Verification items for the finished model (mm, model axes). Give positions to 0.01 mm unless a question says otherwise; leave off trailing zeros. Write each loop counter-clockwise with the first axis right and the second up, starting at its lowest first coordinate (ties: lowest second). Pieces come first, ordered by that corner, then holes. Notation, with made-up numbers: (10, 24) -> (57, 24) arc R25 ccw to (57, 52) -> close; hole circle Ø7 at (8.25, 58). An arc over 180 degrees is marked (long way). Answer as CSV lines item,"result".
```python
from build123d import *

# Parameters (mm, degrees)
BOSS_EXTRUDE1_DEPTH = 6
CUT_EXTRUDE2_DEPTH  = 6
SKETCH4_R           = 1.6
SKETCH4_W           = 18
SKETCH4_H           = 12
CUT_EXTRUDE3_DEPTH  = 10
FILLET1_R           = 2
FILLET2_R           = 2
SKETCH5_R           = 1.1
CUT_EXTRUDE4_DEPTH  = 10
SKETCH6_R           = 22.5
CUT_EXTRUDE5_DEPTH  = 10
FILLET4_R           = 10
FILLET5_R           = 10
FILLET6_R           = 10
FILLET7_R           = 10
FILLET8_R           = 3
SKETCH8_W           = 40
SKETCH8_H           = 10
CUT_EXTRUDE11_DEPTH = 10
FILLET9_R           = 5
CUT_EXTRUDE13_DEPTH = 10
FILLET10_R          = 2


with BuildPart() as part:
    # Sketch1 → Boss-Extrude1 (new body)
    with BuildSketch(Plane.XY):
        Polygon((0, -126.72), (0, 0), (-109.742739168, 63.36), (-137.242739168, 15.728602792), (-55, -126.72), align=None)
        Polygon((-109.742739168, 63.36), (0, 0), (100, 57.735026919), (109.742739168, 63.36), (82.242739168, 110.991397208), (-82.242739168, 110.991397208), align=None)
        Polygon((100, 57.735026919), (0, 0), (0, -126.72), (55, -126.72), (137.242739168, 15.728602792), (109.742739168, 63.36), align=None)
    extrude(amount=BOSS_EXTRUDE1_DEPTH)

    # Sketch3 → Cut-Extrude2 (cut)
    with BuildSketch(Plane.XY.offset(6)):
        Polygon((-109.742739168, 63.36), (-114.742739168, 54.699745962), (-62.78121494, 24.699745962), (-57.78121494, 33.36), align=None)
        Polygon((-104.742739168, 72.020254038), (-109.742739168, 63.36), (-57.78121494, 33.36), (-52.78121494, 42.020254038), align=None)
        Polygon((104.742739168, 72.020254038), (52.78121494, 42.020254038), (57.78121494, 33.36), (62.78121494, 24.699745962), (114.742739168, 54.699745962), align=None)
        Polygon((10, -126.72), (10, -66.72), (0, -66.72), (-10, -66.72), (-10, -126.72), align=None)
    extrude(amount=-CUT_EXTRUDE2_DEPTH, mode=Mode.SUBTRACT)

    # Sketch4 → Cut-Extrude3 (cut)
    with BuildSketch(Plane.XY.offset(6)):
        with Locations((21, -87.47)):
            Circle(SKETCH4_R)
        with Locations((33, -87.47)):
            Circle(SKETCH4_R)
        with Locations((21, -111.47)):
            Circle(SKETCH4_R)
        with Locations((33, -111.47)):
            Circle(SKETCH4_R)
        with Locations((-86.251242069, 25.548466521)):
            Circle(SKETCH4_R)
        with Locations((-92.251242069, 15.156161675)):
            Circle(SKETCH4_R)
        with Locations((-113.03585176, 27.156161675)):
            Circle(SKETCH4_R)
        with Locations((-107.03585176, 37.548466521)):
            Circle(SKETCH4_R)
        with Locations((65.251242069, 61.921533479)):
            Circle(SKETCH4_R)
        with Locations((59.251242069, 72.313838325)):
            Circle(SKETCH4_R)
        with Locations((80.03585176, 84.313838325)):
            Circle(SKETCH4_R)
        with Locations((86.03585176, 73.921533479)):
            Circle(SKETCH4_R)
        Polygon((-111.856909844, 25.898148973), (-101.464604998, 19.898148973), (-110.464604998, 4.309691705), (-120.856909844, 10.309691705), align=None)
        Polygon((69.356909844, 99.510308295), (58.964604998, 93.510308295), (67.964604998, 77.921851027), (78.356909844, 83.921851027), align=None)
        with Locations((42.5, -103.82)):
            Rectangle(SKETCH4_W, SKETCH4_H)
    extrude(amount=-CUT_EXTRUDE3_DEPTH, mode=Mode.SUBTRACT)

    # Fillet1
    fillet1_edges = [part.edges().sort_by_distance(p)[0] for p in [
        (33.5, -109.82, 3),
        (33.5, -97.82, 3),
        (51.5, -97.82, 3),
        (51.5, -109.82, 3),
    ]]
    fillet(fillet1_edges, radius=FILLET1_R)

    # Fillet2
    fillet2_edges = [part.edges().sort_by_distance(p)[0] for p in [
        (-120.856909844, 10.309691705, 3),
        (-111.856909844, 25.898148973, 3),
        (-101.464604998, 19.898148973, 3),
        (-110.464604998, 4.309691705, 3),
    ]]
    fillet(fillet2_edges, radius=FILLET2_R)

    # Sketch5 → Cut-Extrude4 (cut)
    with BuildSketch(Plane.XY.offset(6)):
        with Locations((115.495143903, 45.896542732)):
            Circle(SKETCH5_R)
        with Locations((108.999953375, 42.146542732)):
            Circle(SKETCH5_R)
        with Locations((102.504762847, 38.396542732)):
            Circle(SKETCH5_R)
        with Locations((-18, -122.97)):
            Circle(SKETCH5_R)
        with Locations((-18, -115.47)):
            Circle(SKETCH5_R)
        with Locations((-18, -107.97)):
            Circle(SKETCH5_R)
        with Locations((-97.495143903, 77.073457268)):
            Circle(SKETCH5_R)
        with Locations((-90.999953375, 73.323457268)):
            Circle(SKETCH5_R)
        with Locations((-84.504762847, 69.573457268)):
            Circle(SKETCH5_R)
    extrude(amount=-CUT_EXTRUDE4_DEPTH, mode=Mode.SUBTRACT)

    # Sketch6 → Cut-Extrude5 (cut)
    with BuildSketch(Plane.XY.offset(6)):
        Circle(SKETCH6_R)
    extrude(amount=-CUT_EXTRUDE5_DEPTH, mode=Mode.SUBTRACT)

    # Fillet4
    fillet4_edges = [part.edges().sort_by_distance(p)[0] for p in [
        (-10, -66.72, 3),
        (10, -66.72, 3),
    ]]
    fillet(fillet4_edges, radius=FILLET4_R - 0.0001)  # a hair under: the kernel refuses the full size

    # Fillet5
    fillet5_edges = [part.edges().sort_by_distance(p)[0] for p in [
        (62.78121494, 24.699745962, 3),
        (52.78121494, 42.020254038, 3),
    ]]
    fillet(fillet5_edges, radius=FILLET5_R - 0.0001)  # a hair under: the kernel refuses the full size

    # Fillet6
    fillet6_edges = [part.edges().sort_by_distance(p)[0] for p in [
        (-52.78121494, 42.020254038, 3),
        (-62.78121494, 24.699745962, 3),
    ]]
    fillet(fillet6_edges, radius=FILLET6_R - 0.0001)  # a hair under: the kernel refuses the full size

    # Fillet7
    fillet7_edges = [part.edges().sort_by_distance(p)[0] for p in [
        (55, -126.72, 3),
        (-55, -126.72, 3),
        (-137.242739168, 15.728602792, 3),
        (-82.242739168, 110.991397208, 3),
        (82.242739168, 110.991397208, 3),
        (137.242739168, 15.728602792, 3),
    ]]
    fillet(fillet7_edges, radius=FILLET7_R)

    # Fillet8
    fillet8_edges = [part.edges().sort_by_distance(p)[0] for p in [
        (-114.742739168, 54.699745962, 3),
        (-104.742739168, 72.020254038, 3),
        (104.742739168, 72.020254038, 3),
        (114.742739168, 54.699745962, 3),
        (10, -126.72, 3),
        (-10, -126.72, 3),
    ]]
    fillet(fillet8_edges, radius=FILLET8_R)

    # Sketch8 → Cut-Extrude11 (cut)
    with BuildSketch(Plane.XY.offset(6)):
        with Locations((0, 35)):
            Rectangle(SKETCH8_W, SKETCH8_H)
        with Locations((0, -35)):
            Rectangle(SKETCH8_W, SKETCH8_H)
    extrude(amount=-CUT_EXTRUDE11_DEPTH, mode=Mode.SUBTRACT)

    # Fillet9
    fillet9_edges = [part.edges().sort_by_distance(p)[0] for p in [
        (20, -40, 3),
        (20, -30, 3),
        (-20, -40, 3),
        (-20, -30, 3),
        (20, 30, 3),
        (20, 40, 3),
        (-20, 30, 3),
        (-20, 40, 3),
    ]]
    fillet(fillet9_edges, radius=FILLET9_R - 0.0001)  # a hair under: the kernel refuses the full size

    # Sketch7 → Cut-Extrude13 (cut)
    with BuildSketch(Plane.XY.offset(6)):
        with BuildLine():
            Line((-47.1, 80), (-47.1, -80))
            ThreePointArc((-47.1, -80), (-45, -82.1), (-42.9, -80))
            Line((-42.9, -80), (-42.9, 80))
            ThreePointArc((-42.9, 80), (-45, 82.1), (-47.1, 80))
        make_face()
        with BuildLine():
            Line((42.9, 80), (42.9, -80))
            ThreePointArc((42.9, -80), (45, -82.1), (47.1, -80))
            Line((47.1, -80), (47.1, 80))
            ThreePointArc((47.1, 80), (45, 82.1), (42.9, 80))
        make_face()
        with BuildLine():
            Line((-105, 2.1), (-65, 2.1))
            ThreePointArc((-65, 2.1), (-62.9, 0), (-65, -2.1))
            Line((-65, -2.1), (-105, -2.1))
            ThreePointArc((-105, -2.1), (-107.1, 0), (-105, 2.1))
        make_face()
        with BuildLine():
            Line((65, 2.1), (105, 2.1))
            ThreePointArc((105, 2.1), (107.1, 0), (105, -2.1))
            Line((105, -2.1), (65, -2.1))
            ThreePointArc((65, -2.1), (62.9, 0), (65, 2.1))
        make_face()
    extrude(amount=-CUT_EXTRUDE13_DEPTH, mode=Mode.SUBTRACT)

    # Fillet10
    fillet10_edges = [part.edges().sort_by_distance(p)[0] for p in [
        (69.356909844, 99.510308295, 3),
        (78.356909844, 83.921851027, 3),
        (67.964604998, 77.921851027, 3),
        (58.964604998, 93.510308295, 3),
    ]]
    fillet(fillet10_edges, radius=FILLET10_R)


solid = part.part
```
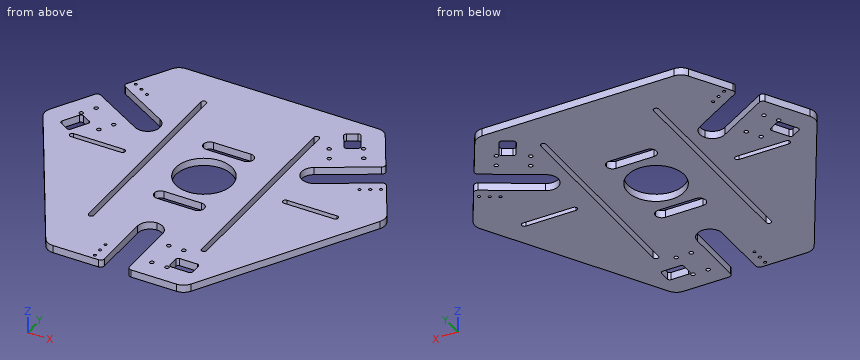
1) Section check B-B (x = -3). Record the boundary of the cut face in (y, z), and give its area (3 significant figures).
Reported:
outline,"(-67.18, 0) -> (-40, 0) -> (-40, 6) -> (-67.18, 6) -> close; (-30, 0) -> (-22.3, 0) -> (-22.3, 6) -> (-30, 6) -> close; (22.3, 0) -> (30, 0) -> (30, 6) -> (22.3, 6) -> close; (40, 0) -> (110.99, 0) -> (110.99, 6) -> (40, 6) -> close"
area,"681 mm²"
2) Section check A-A (y = -62). Record the boundary of the cut face in (x, z), and give its area (3 significant figures).
Reported:
outline,"(-92.37, 0) -> (-47.1, 0) -> (-47.1, 6) -> (-92.37, 6) -> close; (-42.9, 0) -> (42.9, 0) -> (42.9, 6) -> (-42.9, 6) -> close; (47.1, 0) -> (92.37, 0) -> (92.37, 6) -> (47.1, 6) -> close"
area,"1,060 mm²"
3) Depth check by flat-ended pin: pin 1 (3.5 mm diameter, centred on x = 115.5, y = 45.9, fed in from +Z); pin 2 (1.8 mm diameter, centred on x = -94, z = 1.5, fed in from -Y); pin 3 (1.9 mm diameter, centred on x = -86.25, y = 25.55, fed in from +Z); pin 4 (1.5 mm diameter, centred on y = -91, z = 1.5, fed in from +X). Enter the tip coordinate at first touch or a pass-through.
Reported:
pin 1,"z = 6"
pin 2,"y = -60.73"
pin 3,"through"
pin 4,"x = 76.06"
4) Scan lines: line 1 along X through (y, z) = (-107.97, 1.6); line 2 along X through (y, z) = (2.5, 5.25); line 3 along X through (y, z) = (-56, 2.5). Record each from-to range of solid material in increasing order.
Reported:
line 1,"-65.83 to -19.1, -16.9 to -10, 10 to 33.51, 51.49 to 65.83"
line 2,"-129.61 to -47.1, -42.9 to -22.36, 22.36 to 42.9, 47.1 to 129.61"
line 3,"-95.83 to -47.1, -42.9 to 42.9, 47.1 to 95.83"
5) Section check C-C (z = 3.5). State how many separate pieces and enclosed holes the cut face has, and give its area (3 significant figures).
Reported:
separate pieces,"1"
enclosed holes,"31"
area,"39,900 mm²"
